from build123d import *

# Parameters (mm, degrees)
SKETCH1_R               = 4
BOSS_EXTRUDE1_DEPTH     = 10
SKETCH2_R               = 2.5
CUT_EXTRUDE1_DEPTH      = 1
CUT_EXTRUDE1_DEPTH_BACK = 10


with BuildPart() as part:
    # Sketch1 → Boss-Extrude1 (new body)
    with BuildSketch(Plane.XY):
        with BuildLine():
            Line((-70, -100), (70, -100))
            ThreePointArc((70, -100), (91.213203436, -91.213203436), (100, -70))
            Line((100, -70), (100, 70))
            ThreePointArc((100, 70), (91.213203436, 91.213203436), (70, 100))
            Line((70, 100), (-70, 100))
            ThreePointArc((-70, 100), (-91.213203436, 91.213203436), (-100, 70))
            Line((-100, 70), (-100, -70))
            ThreePointArc((-100, -70), (-91.213203436, -91.213203436), (-70, -100))
        make_face()
        with Locations((49.983002612, -3.429415932)):
            Circle(SKETCH1_R, mode=Mode.SUBTRACT)
    extrude(amount=BOSS_EXTRUDE1_DEPTH)

    # Sketch2 → Cut-Extrude1 (cut, two sides)
    with BuildSketch(Plane.XY.offset(10)) as cut_extrude1_sk:
        with Locations((-57.5, 75)):
            Circle(SKETCH2_R)
        with Locations((57.5, 65)):
            Circle(SKETCH2_R)
    extrude(amount=CUT_EXTRUDE1_DEPTH, mode=Mode.SUBTRACT)
    extrude(cut_extrude1_sk.sketch, amount=-CUT_EXTRUDE1_DEPTH_BACK, mode=Mode.SUBTRACT)


solid = part.part
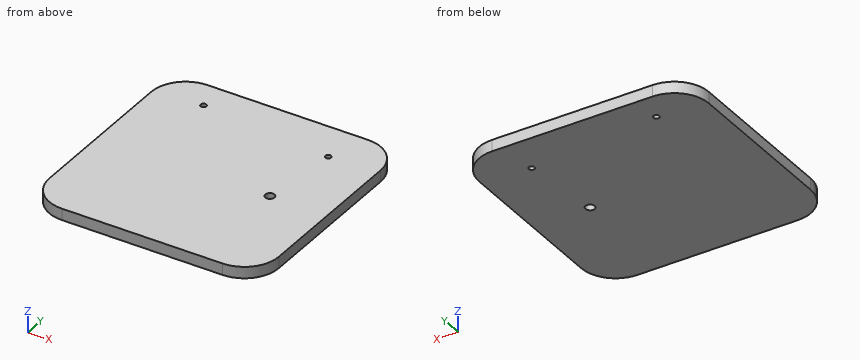
Check sheet for the modelled part. Datum: model origin and axes. Units: mm. Round coordinates to 2 decimals unless told otherwise and drop trailing zeros. Loops run counter-clockwise (first coordinate to the right, second up) from the corner with the lowest first, then second, coordinate; pieces in that order, holes last. Notation, with made-up numbers: M -22.75,80 L 9.25,80 A13 cw 9.25,90 Z; hole C 30,-27 d7. An arc over 180 degrees is marked long. One line per item, written item: value.
(1) Thickness scan on line 1 (Y direction, x = 57.5, z = 3); line 2 (Y direction, x = -57.5, z = 4); line 3 (X direction, y = 71, z = 6.75). Record the ranges inside material, lowest first.
Computed values:
line 1: y = -100 to 62.5, 67.5 to 100
line 2: y = -100 to 72.5, 77.5 to 100
line 3: x = -99.98 to 99.98
(2) Depth check by flat-ended pin: pin 1 Ø10 at (x, y) = (-51.5, 35) entering from -Z; pin 2 Ø4.5 at (x, y) = (57.5, 65) entering from -Z. Enter the tip coordinate at first touch or a pass-through.
Computed values:
pin 1: stops at z = 0
pin 2: passes through
(3) Sectioned sample at C-C, the plane z = 5.25. Record the cut outline in (x, y), then the cut area to 3 significant figures.
Computed values:
outline: M -100,-70 A30 ccw -70,-100 L 70,-100 A30 ccw 100,-70 L 100,70 A30 ccw 70,100 L -70,100 A30 ccw -100,70 Z; hole C -57.5,75 d5; hole C 49.98,-3.43 d8; hole C 57.5,65 d5
area: 39,100 mm^2
(4) Sectioned sample at B-B, the plane y = 65. Record the cut outline in (x, z), then the cut area to 3 significant figures.
Computed values:
outline: M -100,0 L 55,0 L 55,10 L -100,10 Z; M 60,0 L 100,0 L 100,10 L 60,10 Z
area: 1,950 mm^2
(5) Sectioned sample at D-D, the plane x = 86.5. Record the cut outline in (y, z).
Computed values:
outline: M -95.05,0 L 95.05,0 L 95.05,10 L -95.05,10 Z
(6) Sectioned sample at A-A, the plane x = 57.5. Record the cut outline in (y, z).
Computed values:
outline: M -100,0 L 62.5,0 L 62.5,10 L -100,10 Z; M 67.5,0 L 100,0 L 100,10 L 67.5,10 Z
